from build123d import *

# Parameters (mm, degrees)
SKETCH_1_W             = 106
SKETCH_1_H             = 10
EXTRUDE_1_DEPTH        = 7.5
EXTRUDE_2_DEPTH        = 15
PATTERN_LINEAR_1_COUNT = 17
PATTERN_LINEAR_1_PITCH = 6.283185307
SKETCH_3_W             = 10
SKETCH_3_H             = 10
EXTRUDE_1_2_DEPTH      = 18.5
SKETCH_4_R             = 1.4
CUT_EXTRUDE_1_DEPTH    = 119.490505949
FILLET_2_R             = 2
FILLET_3_R             = 2
CHAMFER_1_SIZE         = 0.5


with BuildPart() as part:
    # 草图1 → Extrude 1 (new, symmetric)
    with BuildSketch(Plane.XY):
        with Locations((53, -5)):
            Rectangle(SKETCH_1_W, SKETCH_1_H)
    extrude(amount=EXTRUDE_1_DEPTH, both=True)

    # 草图2 → 拉伸2 (add)
    with BuildSketch(Plane.XY.offset(7.5)):
        Polygon((0, 0), (1.637866054, 4.5), (3.323577771, 4.5), (4.961443825, 0), align=None)
    extrude_2 = extrude(amount=-EXTRUDE_2_DEPTH)

    # 阵列(线性)1: 拉伸2 ×17
    with Locations(*[(i * PATTERN_LINEAR_1_PITCH, 0, 0) for i in range(1, PATTERN_LINEAR_1_COUNT)]):
        add(extrude_2)

    # 草图3 → Extrude 1 2 (add)
    with BuildSketch(Plane.XY.offset(7.5)):
        with Locations((5, -5)):
            Rectangle(SKETCH_3_W, SKETCH_3_H)
    extrude_1_2 = extrude(amount=EXTRUDE_1_2_DEPTH)

    # 镜向1: Extrude 1 2 across plane
    add(extrude_1_2.mirror(Plane.XY))

    # 草图4 → 切除-拉伸1 (cut, through all)
    with BuildSketch(Plane.XY.offset(26)):
        with Locations((5, -5)):
            Circle(SKETCH_4_R)
    extrude(amount=-CUT_EXTRUDE_1_DEPTH, mode=Mode.SUBTRACT)

    # 圆角2
    fillet_2_edges = [part.edges().sort_by_distance(p)[0] for p in [
        (58, -10, 7.5),
        (58, -10, -7.5),
    ]]
    fillet(fillet_2_edges, radius=FILLET_2_R)

    # 圆角3
    fillet_3_edges = [part.edges().sort_by_distance(p)[0] for p in [
        (10, -10, 15.75),
        (10, -10, -15.75),
        (0, -10, 0),
    ]]
    fillet(fillet_3_edges, radius=FILLET_3_R)

    # 倒角1
    chamfer_1_edges = [part.edges().sort_by_distance(p)[0] for p in [
        (3.6, -5, -26),
        (3.6, -5, 26),
    ]]
    chamfer(chamfer_1_edges, length=CHAMFER_1_SIZE)


solid = part.part
Here's how the part is built. I have some questions about the finished solid (model axes, mm). A direction names the side the tool comes from. Round coordinates to 2 decimals unless told otherwise and drop trailing zeros. Write each loop counter-clockwise with the first axis right and the second up, starting at its lowest first coordinate (ties: lowest second). Pieces come first, ordered by that corner, then holes.
1. I need wall thicknesses on L1, parallel to Y at x = 5, z = 9; L2, parallel to Z at x = 14, y = 1.5; L3, parallel to X at y = -3.75, z = -3.5. Which ranges of each line are inside material? Lowest first, please.
2. Will these pins go through, and if not, where does the flat tip stop? pin 1 Ø6 at (x, y) = (54.5, -2) entering from -Z; pin 2 Ø0.7 at (x, z) = (74.5, -3.5) entering from +Y; pin 3 Ø3 at (x, y) = (27.5, 0) entering from +Z.
3. Suppose I cut it at B-B (y = -1.25). List the corners of the cut face in (x, z) for me.
4. Suppose I cut it at A-A (z = 20.5). List the corners of the cut face in (x, y) for me, and give its area (3 significant figures).
5. For faces 1 (the flat face through (88.772, 2.218, 0.105)), 2 (the cylindrical face through (57.69, -9.43, -6.9)), 3 (the flat face through (7.2, -4.9, 26)), which set-ups out of +Z, -Z, +X, -X, +Y, -Y let a thin tool reach every point of the face, with its end or its side?
6. If we mould it in two halves opening along X, with no side actions, what happens to faces 4 (the flat face through (3, 2, -7.5)), 5 (the flat face through (13.374, 2.218, 0.105)), 6 (the cylindrical face through (9.4, -9.43, 15.89))? For each: released by +X, released by -X, zero draft, split by the parting line, or undercut.
Answer sheet:
1. L1: y = -10 to -6.4, -3.6 to 0
1. L2: z = -7.5 to 7.5
1. L3: x = 0 to 4.37, 5.63 to 106
2. pin 1: stops at z = -7.5
2. pin 2: stops at y = 0
2. pin 3: stops at z = 7.5
3. outline: (0, -26) - (10, -26) - (10, -7.5) - (106, -7.5) - (106, 7.5) - (10, 7.5) - (10, 26) - (0, 26) - close
4. outline: (0, -8) arc R2 ccw to (2, -10) - (8, -10) arc R2 ccw to (10, -8) - (10, 0) - (0, 0) - close; hole circle Ø2.8 at (5, -5)
4. area: 92.1 mm2
5. face 1: +Z, -Z, +Y
5. face 2: -Z, +X, -Y
5. face 3: +Z, +X, -X, +Y, -Y
6. face 4: zero draft
6. face 5: undercut
6. face 6: released by +X
